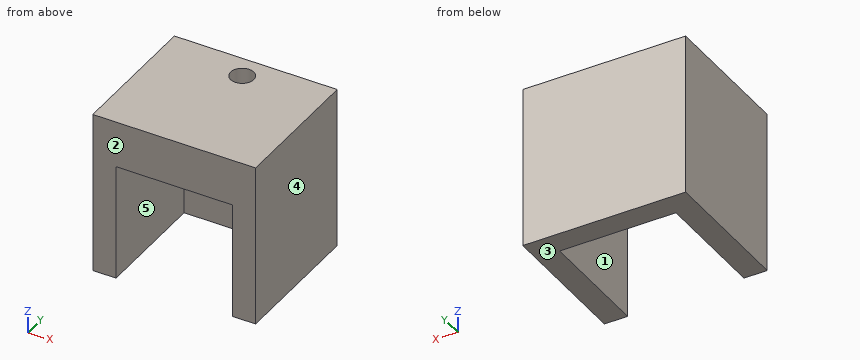
from build123d import *

# Parameters (mm, degrees)
F1_DEPTH = 10
F2_W     = 14
F2_H     = 4.2422189787
F2_H_2   = 7.7577810213
F3_DEPTH = 4
F4_D     = 2
F4_DEPTH = 4.001


with BuildPart() as f1:
    # F0 (on Top) → F1 (new body)
    with BuildSketch(Plane.XY):
        Polygon((7, 6), (-7, 6), (-7, -6), (-5, -6), (-5, 4), (5, 4), (5, -6), (7, -6), align=None)
    extrude(amount=F1_DEPTH)

    # F2 (on face) → F3 (join)
    with BuildSketch(Plane.XY.offset(10)):
        with Locations((0, 3.8788905106)):
            Rectangle(F2_W, F2_H)
        with Locations((0, -2.1211094894)):
            Rectangle(F2_W, F2_H_2)
    extrude(amount=F3_DEPTH)

    # F4 (through all, one way)
    with BuildSketch(Plane(origin=(0, 0, 10), x_dir=(1, 0, 0), z_dir=(0, 0, -1))):
        with Locations((0, -4)):
            Circle(F4_D / 2)
    extrude(amount=-F4_DEPTH, mode=Mode.SUBTRACT)


solid = f1.part
Geometry check sheet. Reference: the model listing, model coordinates, mm. Face numbers are marked on the shaded views. A direction names the side the tool comes from. Coordinates: 2 decimals unless noted, no trailing zeros. Order: outer loops, then holes, each group sorted by start corner. A loop starts at its lowest first (then second) coordinate and runs counter-clockwise, first axis right, second up. Notation, with made-up numbers: (-35.75, 56.5) - (-20.75, 56.5) arc R30 ccw to (-20.75, 83.5) - close; hole circle Ø10 at (-36.75, 79). An arc over 180 degrees is marked (long way). One line per item, written item: value.
(1) Release check for a two-part mould opening along X. For the marked faces 3, 4 and 5 record: +X half, -X half, draft (parallel to the pull), parting line (faces both ways), or undercut.
Data:
face 3: draft
face 4: +X half
face 5: undercut
(2) Sectioned sample at B-B (z = 4.75). Enter the section's corners in (x, y).
Data:
outline: (-7, -6) - (-5, -6) - (-5, 4) - (5, 4) - (5, -6) - (7, -6) - (7, 6) - (-7, 6) - close
(3) Thickness scan on probe 1 along Y at (x, z) = (0, 12.95); probe 2 along X at (y, z) = (-3.25, 9.5); probe 3 along X at (y, z) = (4, 11.75). Record the ranges inside material, lowest first. Write a range as from..to.
Data:
probe 1: y = -6..3, 5..6
probe 2: x = -7..-5, 5..7
probe 3: x = -7..-1, 1..7
(4) Sectioned sample at C-C (y = 2.25). Enter the section's corners in (x, z).
Data:
outline: (-7, 0) - (-5, 0) - (-5, 10) - (5, 10) - (5, 0) - (7, 0) - (7, 14) - (-7, 14) - close
(5) Depth check by flat-ended pin: pin 1 Ø5 at (x, z) = (1, 5) entering from -Y. Enter the tip coordinate at first touch or a pass-through.
Data:
pin 1: stops at y = 4
(6) Sectioned sample at D-D (x = 3.5). Enter the section's corners in (y, z), and give its area (3 significant figures).
Data:
outline: (-6, 10) - (4, 10) - (4, 0) - (6, 0) - (6, 14) - (-6, 14) - close
area: 68.0 mm^2
(7) Sectioned sample at A-A (x = 0). Enter the section's corners in (y, z), and give its area (3 significant figures).
Data:
outline: (-6, 10) - (3, 10) - (3, 14) - (-6, 14) - close; (4, 0) - (6, 0) - (6, 14) - (5, 14) - (5, 10) - (4, 10) - close
area: 60.0 mm^2
(8) Access from +Z, -Z, +X, -X, +Y, -Y to the whole of each face (thin tool, end or side, straight path). Record for the marked faces 1 and 2.
Data:
face 1: -Z, -Y
face 2: +Z, -Z, +X, -X, -Y
